CAD build for the part. Positions are in the model's coordinates, mm. Round coordinates to 2 decimals unless told otherwise and drop trailing zeros. Order: outer loops, then holes, each group sorted by start corner. A loop starts at its lowest first (then second) coordinate and runs counter-clockwise, first axis right, second up. Notation, with made-up numbers: M -17,72 L 37,72 A30 cw 37,98 Z; hole C 26.5,38.5 d5. An arc over 180 degrees is marked long. Put each result on its own line as item: value.
```python
from build123d import *

# Parameters (mm, degrees)
SKETCH1_R                    = 38.1
BOSS_EXTRUDE1_DEPTH          = 1.5875
F_1_4_CLEARANCE_HOLE1_D      = 6.7564
F_1_4_CLEARANCE_HOLE2_D      = 6.7564
F_1_8_0_125_DIAMETER_HOLE1_D = 3.175
F_27_0_144_DIAMETER_HOLE1_D  = 3.6576


with BuildPart() as part:
    # Sketch1 → Boss-Extrude1 (new body, symmetric)
    with BuildSketch(Plane(origin=(0, 0, 0), x_dir=(1, 0, 0), z_dir=(0, 1, 0))):
        Circle(SKETCH1_R)
    extrude(amount=BOSS_EXTRUDE1_DEPTH, both=True)

    # 1/4 Clearance Hole1 (through all)
    with Locations(Plane(origin=(0, 1.5875, 0), x_dir=(1, 0, 0), z_dir=(0, 1, 0))):
        with Locations((-21.59, -17.810706314), (21.59, -17.810706314)):
            Hole(F_1_4_CLEARANCE_HOLE1_D / 2)

    # 1/4 Clearance Hole2 (through all)
    with Locations(Plane(origin=(0, 1.5875, 0), x_dir=(1, 0, 0), z_dir=(0, 1, 0))):
        with Locations((0, 0)):
            Hole(F_1_4_CLEARANCE_HOLE2_D / 2)

    # 1/8 (0.125) Diameter Hole1 (through all)
    with Locations(Plane(origin=(0, 1.5875, 0), x_dir=(1, 0, 0), z_dir=(0, 1, 0))):
        with Locations((0, -31.75), (6.35, -31.75)):
            Hole(F_1_8_0_125_DIAMETER_HOLE1_D / 2)

    # #27 (0.144) Diameter Hole1 (through all)
    with Locations(Plane(origin=(0, 1.5875, 0), x_dir=(1, 0, 0), z_dir=(0, 1, 0))):
        with Locations((-16.51, 7.62), (16.51, 7.62), (16.51, -7.62), (-16.51, -7.62)):
            Hole(F_27_0_144_DIAMETER_HOLE1_D / 2)


solid = part.part
```
Item 1: Pin check, flat tips, straight feed: P1, Ø1.5, axis at x = -6, y = 0, coming from the -Z side; P2, Ø1, axis at x = 27, y = -1, coming from the -Z side. Stop position of each tip, or through.
Answers below:
P1: z = -37.74
P2: z = -27.37
Item 2: Band-saw the part on D-D on x = -16.51. Give the cut face in (y, z).
Answers below:
outline: M -1.59,-34.34 L 1.59,-34.34 L 1.59,-9.45 L -1.59,-9.45 Z; M -1.59,-5.79 L 1.59,-5.79 L 1.59,5.79 L -1.59,5.79 Z; M -1.59,9.45 L 1.59,9.45 L 1.59,34.34 L -1.59,34.34 Z
Item 3: Mould opens along Z. For faces 1 (the cylindrical face through (-30.235, 0.022, 23.183)), 2 (the cylindrical face through (-18.91, -0.02, 19.87)), 3 (the cylindrical face through (-15.059, -0.022, -6.507)), 4 (the flat face through (8, 1.588, -1)) say: pulls with the +Z half, pulls with the -Z half, needs draft (parallel to the pull), parting line crosses it, or undercut.
Answers below:
face 1: parting line crosses it
face 2: undercut
face 3: undercut
face 4: needs draft
Item 4: Band-saw the part on A-A on x = 21.59. Give the cut face in (y, z).
Answers below:
outline: M -1.59,-31.39 L 1.59,-31.39 L 1.59,14.43 L -1.59,14.43 Z; M -1.59,21.19 L 1.59,21.19 L 1.59,31.39 L -1.59,31.39 Z
Item 5: Probe line 1 along Z through (x, y) = (0, 0.4); line 2 along X through (y, z) = (1.15, 20); line 3 along X through (y, z) = (-0.05, 31.75). List the from-to ranges inside material, lowest first. Write a range as [from, to].
Answers below:
line 1: [-38.1, -3.38], [3.38, 30.16], [33.34, 38.1]
line 2: [-32.43, -24.16], [-19.02, 19.02], [24.16, 32.43]
line 3: [-21.06, -1.59], [1.59, 4.76], [7.94, 21.06]
Item 6: Band-saw the part on B-B on z = -7.62. Give the cut face in (x, y).
Answers below:
outline: M -37.33,-1.59 L -18.34,-1.59 L -18.34,1.59 L -37.33,1.59 Z; M -14.68,-1.59 L 14.68,-1.59 L 14.68,1.59 L -14.68,1.59 Z; M 18.34,-1.59 L 37.33,-1.59 L 37.33,1.59 L 18.34,1.59 Z
Item 7: Band-saw the part on C-C on y = -0.6. State how many separate pieces and enclosed holes the cut face has, and give its area (3 significant figures).
Answers below:
separate pieces: 1
enclosed holes: 9
area: 4,390 mm²
